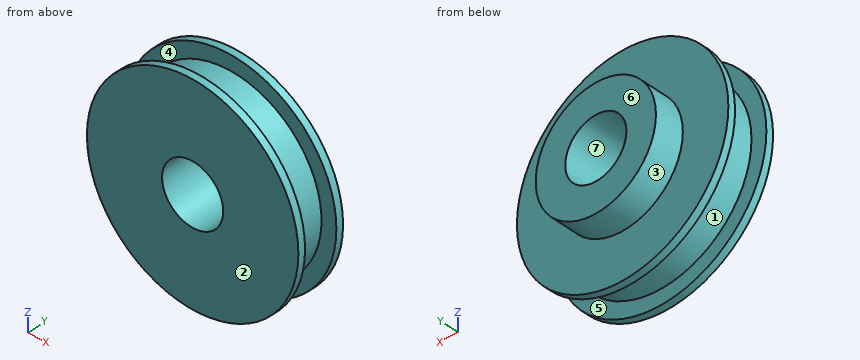
```python
from build123d import *

# Parameters (mm, degrees)
SKETCH2_R          = 6.35
CUT_EXTRUDE1_DEPTH = 17


with BuildPart() as part:
    # Sketch1 → Revolve1 (revolve)
    with BuildSketch(Plane.XY):
        Polygon((0, 0), (0, 16), (-12.5, 16), (-12.5, 10), (-21.971, 10), (-21.971, 8.5), (-18.875, 8.5), (-18.875, 1.5), (-21.971, 1.5), (-21.971, 0), align=None)
    revolve(axis=Axis((0, 0, 0), (0, 1, 0)))

    # Sketch2 → Cut-Extrude1 (cut, through all)
    with BuildSketch(Plane(origin=(0, 16, 0), x_dir=(1, 0, 0), z_dir=(0, 1, 0))):
        Circle(SKETCH2_R)
    extrude(amount=-CUT_EXTRUDE1_DEPTH, mode=Mode.SUBTRACT)


solid = part.part
```
Model file for the job. Use its own axes, mm. Face numbers are marked on the shaded views. A direction names the side the tool comes from. Round coordinates to 2 decimals unless told otherwise and drop trailing zeros. Write each loop counter-clockwise with the first axis right and the second up, starting at its lowest first coordinate (ties: lowest second). Pieces come first, ordered by that corner, then holes. Notation, with made-up numbers: M 32,59.25 L 83,59.25 A20 cw 83,97.25 Z; hole C 55,61.5 d10. An arc over 180 degrees is marked long. Put each result on its own line as item: value.
Item 1: Probe L1, parallel to Y at x = -11.5, z = 16; L2, parallel to Z at x = 0, y = 10.5; L3, parallel to Z at x = 0, y = 5 (3 decimals). List the from-to ranges inside material, lowest first. Write a range as from..to.
Responses:
L1: 0..1.5, 8.5..10
L2: -12.5..-6.35, 6.35..12.5
L3: -18.875..-6.35, 6.35..18.875
Item 2: Cut at A-A (x = 0). List the corners of the cut face in (y, z) (3 decimals), and give its area (3 significant figures).
Responses:
outline: M 0,-21.971 L 1.5,-21.971 L 1.5,-18.875 L 8.5,-18.875 L 8.5,-21.971 L 10,-21.971 L 10,-12.5 L 16,-12.5 L 16,-6.35 L 0,-6.35 Z; M 0,6.35 L 16,6.35 L 16,12.5 L 10,12.5 L 10,21.971 L 8.5,21.971 L 8.5,18.875 L 1.5,18.875 L 1.5,21.971 L 0,21.971 Z
area: 343 mm²
Item 3: Mould opens along Y. For the marked faces 4, 5, 6 and 7 say: +Y half, -Y half, draft (parallel to the pull), parting line (faces both ways), or undercut.
Responses:
face 4: undercut
face 5: undercut
face 6: +Y half
face 7: draft
Item 4: Flat gauge pins, fed straight in: P1, Ø10, axis at x = 0, z = 0, coming from the -Y side; P2, Ø3, axis at x = 16.5, z = -13.5, coming from the +Y side; P3, Ø1.5, axis at x = -4.5, y = 7, coming from the -Z side; P4, Ø3, axis at y = 6, z = -12.5, coming from the -X side. Where does each tip first touch, or does it go through?
Responses:
P1: through
P2: y = 10
P3: z = -18.5
P4: x = -15.34
Item 5: Tool access for the marked faces 1, 2 and 3: list every direction of +Z, -Z, +X, -X, +Y, -Y with a clear straight run to the whole face (end or side of a thin tool).
Responses:
face 1: none
face 2: +Z, -Z, +X, -X, -Y
face 3: +Y
Item 6: Cut at D-D (x = 11). List the corners of the cut face in (y, z).
Responses:
outline: M 0,-19.02 L 1.5,-19.02 L 1.5,-15.34 L 8.5,-15.34 L 8.5,-19.02 L 10,-19.02 L 10,-5.94 L 16,-5.94 L 16,5.94 L 10,5.94 L 10,19.02 L 8.5,19.02 L 8.5,15.34 L 1.5,15.34 L 1.5,19.02 L 0,19.02 Z
Item 7: Cut at B-B (z = 0). List the corners of the cut face in (x, y) (3 decimals), and give its area (3 significant figures).
Responses:
outline: M -21.971,0 L -6.35,0 L -6.35,16 L -12.5,16 L -12.5,10 L -21.971,10 L -21.971,8.5 L -18.875,8.5 L -18.875,1.5 L -21.971,1.5 Z; M 6.35,0 L 21.971,0 L 21.971,1.5 L 18.875,1.5 L 18.875,8.5 L 21.971,8.5 L 21.971,10 L 12.5,10 L 12.5,16 L 6.35,16 Z
area: 343 mm²
Item 8: Cut at C-C (y = 14). List the corners of the cut face in (x, z).
Responses:
outline: C 0,0 d25; hole C 0,0 d12.7
